from build123d import *
from build123d.topology import SkipClean

# Parameters (mm, degrees)
SKETCH1_R                                        = 5.5
SKETCH1_R_2                                      = 3.5
BOSS_EXTRUDE1_DLUGOSC_CALKOWITA_DEPTH            = 50
BOSS_EXTRUDE2_PRZEDLUZENIE_DO_MONTAZU_DEPTH      = 8
BOSS_EXTRUDE2_PRZEDLUZENIE_DO_MONTAZU_DEPTH_BACK = 58


with BuildPart() as part:
    # Sketch1 → Boss-Extrude1 dlugosc calkowita (new body)
    with BuildSketch(Plane.XY):
        Circle(SKETCH1_R)
        Circle(SKETCH1_R_2, mode=Mode.SUBTRACT)
    extrude(amount=BOSS_EXTRUDE1_DLUGOSC_CALKOWITA_DEPTH)

    # Sketch2 → Boss-Extrude2 przedluzenie do montazu (add, two sides: drawn at the far end of the back side and taken through both)
    with SkipClean():  # the faces are left unmerged after this step: merging them gives an invalid solid
        with BuildSketch(Plane(origin=(0, 0, 0), x_dir=(-1, 0, 0), z_dir=(0, 0, -1)).offset(-BOSS_EXTRUDE2_PRZEDLUZENIE_DO_MONTAZU_DEPTH_BACK)):
            with BuildLine():
                Line((0, 5.5), (0, 3.5))
                ThreePointArc((0, 3.5), (3.5, 0), (0, -3.5))
                Line((0, -3.5), (0, -5.5))
                ThreePointArc((0, -5.5), (5.5, 0), (0, 5.5))
            make_face()
        extrude(amount=BOSS_EXTRUDE2_PRZEDLUZENIE_DO_MONTAZU_DEPTH + BOSS_EXTRUDE2_PRZEDLUZENIE_DO_MONTAZU_DEPTH_BACK)
    add(part.part.scale(1), mode=Mode.REPLACE)  # the faces are merged on a copy


solid = part.part
Input: part model. Units: mm. Frame: model coordinates. A direction names the side the tool comes from. Round coordinates to 2 decimals unless told otherwise and drop trailing zeros. Loops run counter-clockwise (first coordinate to the right, second up) from the corner with the lowest first, then second, coordinate; pieces in that order, holes last. Notation, with made-up numbers: M -14,37 L 2,37 A17 cw 2,61 Z; hole C 69.5,66.25 d10. An arc over 180 degrees is marked long. Answer as CSV lines item,"result". Start each with the question number.
(1) Section C-C, the plane z = 36. Output: boundary loops of the cut face in (x, y).
(2) First-contact query: pin 1 (2 mm diameter, centred on y = -5, z = 54, fed in from +X); pin 2 (1 mm diameter, centred on y = -2.5, z = 5, fed in from -X); pin 3 (4 mm diameter, centred on x = 2, z = 46, fed in from +Y); pin 4 (4.5 mm diameter, centred on x = 3.5, y = -2, fed in from +Z). Flat tips, straight axial feed; report the tip coordinate or a pass-through.
(3) Section D-D, the plane y = 4.75. Output: boundary loops of the cut face in (x, z).
(4) Section B-B, the plane y = 2.25. Output: boundary loops of the cut face in (x, z).
(5) Section A-A, the plane x = -2. Output: boundary loops of the cut face in (y, z).
(6) Line query: line 1 (X direction, y = -0.25, z = 40.5); line 2 (Z direction, x = 3.75, y = 2.5); line 3 (X direction, y = 1, z = 27.5). Output: solid intervals per line, ascending. Write a range as [from, to].
(7) Draft query along Z for faces 4 (the flat face through (4, 0, 50)), 5 (the flat face through (4, 0, 0)), 6 (the flat face through (0, -4, -4)). Return one class per face: released by +Z, released by -Z, zero draft, split by the parting line, or undercut.
(8) Reachability of faces 1 (the flat face through (-4, 0, 58)), 2 (the flat face through (0, 5, -4)), 3 (the flat face through (0, 5, 54)) from +Z, -Z, +X, -X, +Y, -Y: full face, straight path, thin tool, end or side. Return the list, or none.
Values found:
1,outline,"C 0,0 d11; hole C 0,0 d7"
2,pin 1,"stops at x = 0"
2,pin 2,"stops at x = -5.12"
2,pin 3,"stops at y = 5.5"
2,pin 4,"stops at z = 50"
3,outline,"M -2.77,-8 L 0,-8 L 0,0 L 2.77,0 L 2.77,50 L 0,50 L 0,58 L -2.77,58 Z"
4,outline,"M -5.02,-8 L -2.68,-8 L -2.68,58 L -5.02,58 Z; M 2.68,0 L 5.02,0 L 5.02,50 L 2.68,50 Z"
5,outline,"M -5.12,-8 L -2.87,-8 L -2.87,58 L -5.12,58 Z; M 2.87,-8 L 5.12,-8 L 5.12,58 L 2.87,58 Z"
6,line 1,"x = [-5.49, -3.49], [3.49, 5.49]"
6,line 2,"z = [0, 50]"
6,line 3,"x = [-5.41, -3.35], [3.35, 5.41]"
7,face 4,"released by +Z"
7,face 5,"released by -Z"
7,face 6,"zero draft"
8,face 1,"+Z, +X, -X, +Y, -Y"
8,face 2,"-Z, +X, +Y, -Y"
8,face 3,"+Z, +X, +Y, -Y"
